Could you check a few things on this model? Use its own coordinates, in mm. A direction names the side the tool comes from. Give positions to 0.01 mm unless a question says otherwise; leave off trailing zeros. Loops run counter-clockwise (first coordinate to the right, second up) from the corner with the lowest first, then second, coordinate; pieces in that order, holes last. Notation, with made-up numbers: M -21,35 L 7,35 A23 cw 7,53 Z; hole C 13,69 d8. An arc over 180 degrees is marked long. Return JSON: item names as keys, results as strings. Group by question number.
1. If we mould it in two halves opening along Z, with no side actions, what happens to faces 4 (the flat face through (-13, 0, -15)), 5 (the cylindrical face through (-15.085, -0.21, -1.302)), 6 (the flat face through (0, 11, -12)), 7 (the conical face through (15.1, 5.27, 2.74))? For each: +Z half, -Z half, draft (parallel to the pull), parting line (faces both ways), or undercut.
2. Please list where these lines run through material, in increasing order: line 1 (Z direction, x = -21, y = 4.5); line 2 (Z direction, x = -30, y = -10.25); line 3 (X direction, y = 7, z = 0).
3. For pin 1 (7.5 mm diameter, centred on y = 7, z = -9, fed in from +X); pin 2 (5 mm diameter, centred on x = 8, z = 1.5, fed in from -Y); pin 3 (7.5 mm diameter, centred on y = -9.5, z = 8, fed in from +X), each with a flat end and sliding along its axis, tell me the tip position at first contact or that it passes through.
4. For faces 1 (the flat face through (0, -12, 11)), 2 (the flat face through (0, 12, 12)), 3 (the flat face through (0, -11, -12)), which set-ups out of +Z, -Z, +X, -X, +Y, -Y let a thin tool reach every point of the face, with its end or its side?
5. If we section it at A-A (x = 20): Write out the boundary of the cut face in (y, z).
```python
from build123d import *

# Parameters (mm, degrees)
BOSS_EXTRUDE2_DEPTH      = 15
BOSS_EXTRUDE2_DEPTH_BACK = 15
SKETCH1_R                = 10


with BuildPart() as part:
    # Sketch1 → Boss-Extrude2 (new, two sides: drawn at the far end of the back side and taken through both)
    with BuildSketch(Plane(origin=(0, 0, 0), x_dir=(1, 0, 0), z_dir=(0, 1, 0)).offset(-BOSS_EXTRUDE2_DEPTH_BACK)):
        with BuildLine():
            Line((-25, 15), (0, 15))
            Line((0, 15), (0, -15))
            Line((0, -15), (-25, -15))
            ThreePointArc((-25, -15), (-40, 0), (-25, 15))
        make_face()
        with Locations(Location((-25, 0, 0), (0, 0, 270))):
            Circle(SKETCH1_R, mode=Mode.SUBTRACT)
    extrude(amount=BOSS_EXTRUDE2_DEPTH + BOSS_EXTRUDE2_DEPTH_BACK)

    # Sketch1_4 → Revolve2 (revolve)
    with BuildSketch(Plane(origin=(0, 0, 0), x_dir=(1, 0, 0), z_dir=(0, 1, 0)), mode=Mode.PRIVATE) as revolve2_sk:
        Polygon((25, 0), (0, 15), (0, 0), align=None)
    revolve(revolve2_sk.sketch.rotate(Axis((0, 0, 0), (1, 0, 0)), 180), axis=Axis((0, 0, 0), (1, 0, 0)))


solid = part.part
```
Answer:
{
 "1": {"face 4": "-Z half", "face 5": "undercut", "face 6": "draft", "face 7": "parting line"},
 "2": {"line 1": "z = -15 to -9.17, 9.17 to 15", "line 2": "z = -14.14 to -8.66, 8.66 to 14.14", "line 3": "x = -40 to -35, -15 to 13.33"},
 "3": {"pin 1": "stops at x = 12.25", "pin 2": "stops at y = -11.63", "pin 3": "stops at x = 10.55"},
 "4": {"face 1": "+Z, +X, -Y", "face 2": "+Z, +X, +Y", "face 3": "-Z, +X, -Y"},
 "5": {"outline": "C 0,0 d6"}
}
